Read the model definition and answer for the solid it produces. Units are mm, in the model's axes. Face numbers are marked on the shaded views. A direction names the side the tool comes from. Round coordinates to 2 decimals unless told otherwise and drop trailing zeros. Order: outer loops, then holes, each group sorted by start corner. A loop starts at its lowest first (then second) coordinate and runs counter-clockwise, first axis right, second up. Notation, with made-up numbers: (43.25, 38.5) -> (59.25, 38.5) arc R20 cw to (59.25, 61.5) -> close; hole circle Ø7 at (-35, -13.5). An arc over 180 degrees is marked (long way). Use a Markdown table: item, result. Add a question column.
1. Consider L1, parallel to Y at x = 43, z = 15; L2, parallel to X at y = 28, z = 48; L3, parallel to X at y = 44.5, z = 46.5. Determine where each line is inside the solid, lowest interval first. Write a range as [from, to].
2. The mould has two halves that part along X. Classify the marked faces 4, 5, 6 and 7: +X half, -X half, draft (parallel to the pull), parting line (faces both ways), or undercut.
3. Section D-D, the plane y = 21.5 is taken. Give the vertices of the cut face in (x, z).
4. For the marked faces 1, 2 and 3, determine the directions among +Z, -Z, +X, -X, +Y, -Y from which every point of the face is accessible in a straight line to the end or side of a thin tool.
5. Section A-A, the plane y = 12.5 is taken. Give the vertices of the cut face in (x, z), then the cut area to 3 significant figures.
6. Section B-B, the plane x = 15.5 is taken. Give the vertices of the cut face in (y, z).
7. Section C-C, the plane z = 20.5 is taken. Give the vertices of the cut face in (x, y) (3 decimals).
8. Given pin 1 (7.5 mm diameter, centred on x = 43.5, z = 14, fed in from +Y), flat-ended and moving along its own axis, determine where the tip first touches the part or whether it passes through.
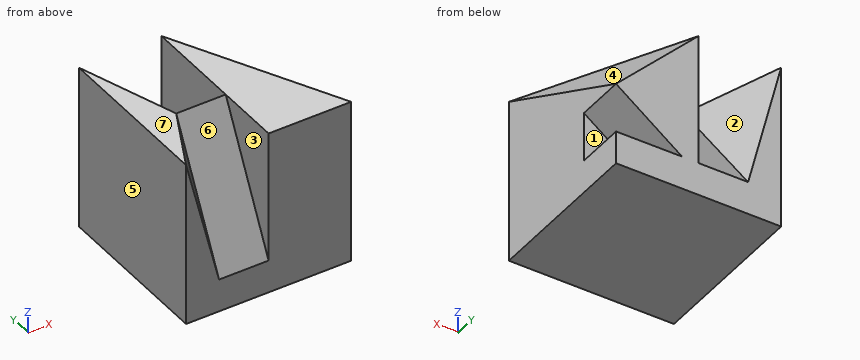
```python
from build123d import *

# Parameters (mm, degrees)
F0_W      = 50
F0_H      = 50
F1_DEPTH  = 50
F11_W     = 15
F11_H     = 20
F14_W     = 15
F14_H     = 30
F18_DEPTH = 15


with BuildPart() as f1:
    # F0 (on Top) → F1 (new body)
    with BuildSketch(Plane.XY):
        with Locations((25, 25)):
            Rectangle(F0_W, F0_H)
    extrude(amount=F1_DEPTH)

    # F4: sweep along a path in F3
    with BuildLine(Plane(origin=(0, 0, 0), x_dir=(0, -1, 0), z_dir=(-1, 0, 0))) as f4_path:
        Line((-20, 50), (-50, 10))
    # F2 (on face) → F4 (sweep, cut)
    with BuildSketch(Plane.XY.offset(50)):
        Polygon((10, 50), (0, 50), (10, 20), align=None)
    sweep(path=f4_path.line, mode=Mode.SUBTRACT)

    # F7: sweep along a path in F6
    with BuildLine(Plane(origin=(0, 0, 0), x_dir=(0, -1, 0), z_dir=(-1, 0, 0))) as f7_path:
        Line((-20, 50), (0, 10))
    # F5 (on face) → F7 (sweep, cut)
    with BuildSketch(Plane.XY.offset(50)):
        Polygon((10, 0), (10, 20), (0, 0), align=None)
    sweep(path=f7_path.line, mode=Mode.SUBTRACT)

    # F10: sweep along a path in F9
    with BuildLine(Plane.YZ.offset(50)) as f10_path:
        Line((0, 50), (50, 25))
    # F8 (on face) → F10 (sweep, cut)
    with BuildSketch(Plane.XY.offset(50)):
        Polygon((50, 50), (25, 50), (50, 0), align=None)
    sweep(path=f10_path.line, mode=Mode.SUBTRACT)

    # F13: sweep along a path in F12
    with BuildLine(Plane(origin=(0, 0, 0), x_dir=(0, -1, 0), z_dir=(-1, 0, 0))) as f13_path:
        Line((-20, 50), (0, 10))
    # F11 (on face) → F13 (sweep, cut)
    with BuildSketch(Plane.XY.offset(50)):
        with Locations((17.5, 10)):
            Rectangle(F11_W, F11_H)
    sweep(path=f13_path.line, mode=Mode.SUBTRACT)

    # F16: sweep along a path in F15
    with BuildLine(Plane(origin=(0, 0, 0), x_dir=(0, -1, 0), z_dir=(-1, 0, 0))) as f16_path:
        Line((-20, 50), (-50, 10))
    # F14 (on face) → F16 (sweep, cut)
    with BuildSketch(Plane.XY.offset(50)):
        with Locations((17.5, 35)):
            Rectangle(F14_W, F14_H)
    sweep(path=f16_path.line, mode=Mode.SUBTRACT)

    # F17 (on face) → F18 (cut)
    with BuildSketch(Plane(origin=(0, 50, 0), x_dir=(-1, 0, 0), z_dir=(0, 1, 0))):
        Polygon((-30.000045, 10.042553), (-50, 25), (-50, 10), align=None)
    extrude(amount=-F18_DEPTH, mode=Mode.SUBTRACT)


solid = f1.part
```
Verdict:
| question | item | result |
|---|---|---|
| 1 | L1 | y = [0, 35] |
| 1 | L2 | x = [0, 7.83], [25, 38] |
| 1 | L3 | x = [0, 2.71], [25, 31.25] |
| 2 | face 4 | +X half |
| 2 | face 5 | -X half |
| 2 | face 6 | undercut |
| 2 | face 7 | draft |
| 3 | outline | (0, 0) -> (50, 0) -> (50, 39.25) -> (39.25, 50) -> (25, 50) -> (25, 48) -> (10, 48) -> (9.5, 50) -> (0, 50) -> close |
| 4 | face 1 | +X, +Y |
| 4 | face 2 | +Z, +Y |
| 4 | face 3 | +Z, -Y |
| 5 | outline | (0, 0) -> (50, 0) -> (50, 43.75) -> (43.75, 50) -> (25, 50) -> (25, 35) -> (10, 35) -> (6.25, 50) -> (0, 50) -> close |
| 5 | area | 2,230 mm2 |
| 6 | outline | (0, 0) -> (50, 0) -> (50, 10) -> (20, 50) -> (0, 10) -> close |
| 7 | outline | (0, 0) -> (7.375, 0) -> (10, 5.25) -> (25, 5.25) -> (25, 0) -> (50, 0) -> (50, 35) -> (43.983, 35) -> (43.983, 50) -> (25, 50) -> (25, 42.125) -> (10, 42.125) -> (7.375, 50) -> (0, 50) -> close |
| 8 | pin 1 | stops at y = 35 |
